Check sheet for the modelled part. Datum: model origin and axes. Units: mm. A direction names the side the tool comes from. Round coordinates to 2 decimals unless told otherwise and drop trailing zeros. Order: outer loops, then holes, each group sorted by start corner. A loop starts at its lowest first (then second) coordinate and runs counter-clockwise, first axis right, second up. Notation, with made-up numbers: (25.25, -15.75) -> (84.25, -15.75) arc R17 cw to (84.25, 15.25) -> close; hole circle Ø10 at (-39, 42.25). An arc over 180 degrees is marked (long way). Answer in a Markdown table with one row per item.
```python
from build123d import *

# Parameters (mm, degrees)
F0_W      = 78
F0_H      = 42
F1_DEPTH  = 2
F2_W      = 2
F2_H      = 4
F2_W_2    = 4
F2_H_2    = 2
F3_DEPTH  = 23.5
F5_DEPTH  = 13.5
F6_W      = 1
F6_H      = 5.3
F6_H_2    = 7.8
F7_DEPTH  = 2.5
F8_R      = 2
F9_W      = 4
F9_H      = 0.8
F10_DEPTH = 1
F11_W     = 4
F11_H     = 0.8
F12_DEPTH = 1
F13_W     = 4
F13_H     = 0.8
F14_DEPTH = 1
F15_W     = 4
F15_H     = 0.8
F16_DEPTH = 1


with BuildPart() as f1:
    # F0 (on Top) → F1 (new body)
    with BuildSketch(Plane.XY):
        with Locations((39, 21)):
            Rectangle(F0_W, F0_H)
    extrude(amount=F1_DEPTH)

    # F2 (on face) → F3 (join)
    with BuildSketch(Plane(origin=(0, 0, 0), x_dir=(1, 0, 0), z_dir=(0, 0, -1))):
        with Locations((0, -32.5)):
            Rectangle(F2_W, F2_H)
        with Locations((12.5, 0)):
            Rectangle(F2_W_2, F2_H_2)
        with Locations((78, -6.5)):
            Rectangle(F2_W, F2_H)
        with Locations((0, -9.5)):
            Rectangle(F2_W, F2_H)
    extrude(amount=-F3_DEPTH)

    # F4 (on face) → F5 (join)
    with BuildSketch(Plane.XY.offset(2)):
        Polygon((26.25, 0), (40.75, 0), (40.75, 1.1), (41.45, 1.1), (41.45, 1.9), (40.75, 1.9), (40.75, 3), (26.25, 3), (26.25, 1.9), (25.55, 1.9), (25.55, 1.1), (26.25, 1.1), align=None)
    extrude(amount=F5_DEPTH)

    # F6 (on face) → F7 (join)
    with BuildSketch(Plane.XY.offset(2)):
        with Locations((0.5, 21.75)):
            Rectangle(F6_W, F6_H)
        with Locations((77.5, 21.3)):
            Rectangle(F6_W, F6_H_2)
    extrude(amount=F7_DEPTH)

    # F8
    f8_edges = [f1.edges().sort_by_distance(p)[0] for p in [
        (78, 42, 1),
        (78, 0, 1),
        (0, 42, 1),
        (0, 0, 1),
    ]]
    fillet(f8_edges, radius=F8_R)

    # F9 (on face) → F10 (join)
    with BuildSketch(Plane(origin=(0, 1, 0), x_dir=(-1, 0, 0), z_dir=(0, 1, 0))):
        with Locations((-12.5, 23.1)):
            Rectangle(F9_W, F9_H)
    extrude(amount=F10_DEPTH)

    # F11 (on face) → F12 (join)
    with BuildSketch(Plane(origin=(77, 0, 0), x_dir=(0, -1, 0), z_dir=(-1, 0, 0))):
        with Locations((-6.5, 23.1)):
            Rectangle(F11_W, F11_H)
    extrude(amount=F12_DEPTH)

    # F13 (on face) → F14 (join)
    with BuildSketch(Plane.YZ.offset(1)):
        with Locations((32.5, 23.1)):
            Rectangle(F13_W, F13_H)
    extrude(amount=F14_DEPTH)

    # F15 (on face) → F16 (join)
    with BuildSketch(Plane.YZ.offset(1)):
        with Locations((9.5, 23.1)):
            Rectangle(F15_W, F15_H)
    extrude(amount=F16_DEPTH)


solid = f1.part
```
(1) Section check A-A on z = 13.5. Record the boundary of the cut face in (x, y).
Solutions:
| item | result |
|---|---|
| outline | (-1, 7.5) -> (1, 7.5) -> (1, 11.5) -> (-1, 11.5) -> close; (-1, 30.5) -> (1, 30.5) -> (1, 34.5) -> (-1, 34.5) -> close; (10.5, -1) -> (14.5, -1) -> (14.5, 1) -> (10.5, 1) -> close; (25.55, 1.1) -> (26.25, 1.1) -> (26.25, 0) -> (40.75, 0) -> (40.75, 1.1) -> (41.45, 1.1) -> (41.45, 1.9) -> (40.75, 1.9) -> (40.75, 3) -> (26.25, 3) -> (26.25, 1.9) -> (25.55, 1.9) -> close; (77, 4.5) -> (79, 4.5) -> (79, 8.5) -> (77, 8.5) -> close |
(2) Scan lines: probe 1 along Z at (x, y) = (6, 11); probe 2 along X at (y, z) = (7, 8); probe 3 along X at (y, z) = (33.5, 16.5). Record each from-to range of solid material in increasing order. Write a range as from..to.
Solutions:
| item | result |
|---|---|
| probe 1 | 0..2 |
| probe 2 | 77..79 |
| probe 3 | -1..1 |
(3) Draft check along X on faces 1 (the flat face through (1, 22, 3)), 2 (the cylindrical face through (77.4, 41.43, 1.01)), 3 (the flat face through (38, 20, 0)). Enter one of: pulls with the +X half, pulls with the -X half, needs draft (parallel to the pull), parting line crosses it, or undercut.
Solutions:
| item | result |
|---|---|
| face 1 | undercut |
| face 2 | pulls with the +X half |
| face 3 | needs draft |
(4) Section check C-C on x = 27.5. Record the boundary of the cut face in (y, z).
Solutions:
| item | result |
|---|---|
| outline | (0, 0) -> (42, 0) -> (42, 2) -> (3, 2) -> (3, 15.5) -> (0, 15.5) -> close |
(5) Tool access check on faces 4 (the flat face through (1, 10, 12)), 5 (the flat face through (12, 1, 12)), 6 (the flat face through (77, 21, 3)), 7 (the flat face through (38, 0, 6)). Record the directions out of +Z, -Z, +X, -X, +Y, -Y that give a thin tool (end or side, any length) a straight path to the whole face; none if there is none.
Solutions:
| item | result |
|---|---|
| face 4 | +Y, -Y |
| face 5 | -X, +Y |
| face 6 | +Z, +Y, -Y |
| face 7 | +Z, -Z, +X, -Y |
(6) Section check D-D on z = 3.25. Give the number of separate pieces and of enclosed holes in the cut face, plus the area to 3 significant figures.
Solutions:
| item | result |
|---|---|
| separate pieces | 7 |
| enclosed holes | 0 |
| area | 89.7 mm^2 |
(7) Depth check by flat-ended pin: pin 1 Ø2 at (y, z) = (38, 1) entering from -X; pin 2 Ø12 at (x, y) = (56.5, 21.5) entering from +Z; pin 3 Ø1.5 at (x, z) = (77, 15.5) entering from +Y. Enter the tip coordinate at first touch or a pass-through.
Solutions:
| item | result |
|---|---|
| pin 1 | x = 0 |
| pin 2 | z = 2 |
| pin 3 | y = 8.5 |
(8) Section check B-B on y = 5.5. Record the boundary of the cut face in (x, z).
Solutions:
| item | result |
|---|---|
| outline | (0, 0) -> (79, 0) -> (79, 23.5) -> (76, 23.5) -> (76, 22.7) -> (77, 22.7) -> (77, 2) -> (0, 2) -> close |
